Source: CAD feature listing. Evaluate the final solid. Frame: model axes, mm. A direction names the side the tool comes from. Give positions to 0.01 mm unless a question says otherwise; leave off trailing zeros. Order: outer loops, then holes, each group sorted by start corner. A loop starts at its lowest first (then second) coordinate and runs counter-clockwise, first axis right, second up. Notation, with made-up numbers: M 23,-4 L 79,-4 A17 cw 79,9 Z; hole C -35,25 d9. An arc over 180 degrees is marked long. Use CSV: the item, a comma, the result in double quotes. Start each with the question number.
1. Section query B-B, the plane x = 20. Return the cut outline in (y, z), plus the area to 3 significant figures.
2. Reachability of faces 5 (the flat face through (-26, 2, 0)), 6 (the flat face through (0, 28.8, 30)) from +Z, -Z, +X, -X, +Y, -Y: full face, straight path, thin tool, end or side. Return the list, or none.
3. Section query A-A, the plane y = 0. Return the cut outline in (x, z), plus the area to 3 significant figures.
4. Mould query, pull axis X, two halves, no side actions, for faces 1 (the flat face through (-7, 26, 30)), 2 (the flat face through (7, 26, 30)), 3 (the flat face through (-26, 2, 60)), 4 (the cylindrical face through (105.874, -33.341, 29.58)). Classes: released by +X, released by -X, zero draft, split by the parting line, or undercut.
5. Section query D-D, the plane y = 34.5. Return the cut outline in (x, z).
6. Section query C-C, the plane z = 27. Return the cut outline in (x, y), plus the area to 3 significant figures.
7. Line query: line 1 along Y through (x, z) = (0, 24.5); line 2 along Y through (x, z) = (42, 50); line 3 along X through (y, z) = (17, 10.5). Output: solid intervals per line, ascending. Write a range as [from, to].
8. Pin query (flat end, axial travel): P1, Ø1.5, axis at x = -83.5, z = 41.5, coming from the -Y side; P2, Ø2.5, axis at y = 27, z = 41, coming from the +X side; P3, Ø12, axis at x = 12.5, z = 14.5, coming from the +Y side. Return the tip coordinate at first contact, or that it passes through.
Autodesk Inventor part; units mm, degrees
sketch "スケッチ1" plane through (0, 0, 0) normal (0, 0, 1) x (1, 0, 0)
  circle A0 centre (0, 0) radius 111
  arc A1 (-7, 24) -> (7, 24) centre (0, 0) ccw
  line L0 (0, 25) -> (0, 28.8)
  line L1 (0, 28.8) -> (0, 20)
  line L2 (0, 20) -> (-7, 20)
  line L3 (-7, 24) -> (-7, 28.8)
  line L4 (-7, 28.8) -> (7, 28.8)
  line L5 (7, 28.8) -> (7, 24)
  line L6 (7, 20) -> (0, 20)
  dimension "d0" = 222
  dimension "d1" = 50
  dimension "d2" = 3.8
  dimension "d3" = 8.8
  dimension "d4" = 7
  dimension "d5" = 14
extrude "押し出し1" add sketch "スケッチ1" along normal blind 60
properties part number "gear4"
Result set:
1,outline,"M -109.18,0 L -15,0 L -15,60 L -109.18,60 Z; M 15,0 L 109.18,0 L 109.18,60 L 15,60 Z"
1,area,"11,300 mm2"
2,face 5,"-Z, +X, -X, +Y, -Y"
2,face 6,"+Z, -Z"
3,outline,"M -111,0 L -25,0 L -25,60 L -111,60 Z; M 25,0 L 111,0 L 111,60 L 25,60 Z"
3,area,"10,300 mm2"
4,face 1,"undercut"
4,face 2,"undercut"
4,face 3,"zero draft"
4,face 4,"split by the parting line"
5,outline,"M -105.5,0 L 105.5,0 L 105.5,60 L -105.5,60 Z"
6,outline,"C 0,0 d222; hole M -7,24 A25 ccw long 7,24 L 7,28.8 L -7,28.8 Z"
6,area,"36,700 mm2"
7,line 1,"[-111, -25], [28.8, 111]"
7,line 2,"[-102.75, 102.75]"
7,line 3,"[-109.69, -18.33], [18.33, 109.69]"
8,P1,"y = -73.98"
8,P2,"x = 107.97"
8,P3,"y = 110.81"
